Check sheet for the modelled part. Datum: model origin and axes. Units: mm. A direction names the side the tool comes from. Round coordinates to 2 decimals unless told otherwise and drop trailing zeros. Write each loop counter-clockwise with the first axis right and the second up, starting at its lowest first coordinate (ties: lowest second). Pieces come first, ordered by that corner, then holes. Notation, with made-up numbers: M 0,68.5 L 7,68.5 A20 ccw 7,95.5 Z; hole C -1,85.25 d10. An arc over 180 degrees is marked long. Put each result on its own line as item: value.
```python
from build123d import *

# Parameters (mm, degrees)
SKETCH1_W           = 30
SKETCH1_H           = 12
BOSS_EXTRUDE1_DEPTH = 3
SKETCH3_W           = 5
SKETCH3_H           = 3
BOSS_EXTRUDE2_DEPTH = 3
SKETCH4_W           = 3
SKETCH4_H           = 3
CUT_EXTRUDE1_DEPTH  = 10


with BuildPart() as part:
    # Sketch1 → Boss-Extrude1 (new body)
    with BuildSketch(Plane(origin=(0, 0, 0), x_dir=(0, 0, -1), z_dir=(1, 0, 0))):
        Rectangle(SKETCH1_W, SKETCH1_H)
    extrude(amount=BOSS_EXTRUDE1_DEPTH)

    # Sketch3 → Boss-Extrude2 (add)
    with BuildSketch(Plane(origin=(3, 0, 0), x_dir=(0, 0, -1), z_dir=(1, 0, 0))):
        with Locations((-10, 7.5)):
            Rectangle(SKETCH3_W, SKETCH3_H)
        with Locations((0, 7.5)):
            Rectangle(SKETCH3_W, SKETCH3_H)
        with Locations((10, 7.5)):
            Rectangle(SKETCH3_W, SKETCH3_H)
        with Locations((10, -7.5)):
            Rectangle(SKETCH3_W, SKETCH3_H)
        with Locations((0, -7.5)):
            Rectangle(SKETCH3_W, SKETCH3_H)
        with Locations((-10, -7.5)):
            Rectangle(SKETCH3_W, SKETCH3_H)
    extrude(amount=-BOSS_EXTRUDE2_DEPTH)

    # Sketch4 → Cut-Extrude1 (cut)
    with BuildSketch(Plane(origin=(3, 0, 0), x_dir=(0, 0, -1), z_dir=(1, 0, 0))):
        with Locations((-5, -1.5)):
            Rectangle(SKETCH4_W, SKETCH4_H)
        with Locations((5, -1.5)):
            Rectangle(SKETCH4_W, SKETCH4_H)
    extrude(amount=-CUT_EXTRUDE1_DEPTH, mode=Mode.SUBTRACT)


solid = part.part
```
1. Cross-section at D-D (z = 13.25). Enter the section's corners in (x, y), then the cut area to 3 significant figures.
Computed values:
outline: M 0,-6 L 3,-6 L 3,6 L 0,6 Z
area: 36.0 mm2
2. Access from +Z, -Z, +X, -X, +Y, -Y to the whole of each face (thin tool, end or side, straight path). Record for faces 4 (the flat face through (2, 7, 2.5)), 5 (the flat face through (2, -8, -2.5)), 6 (the flat face through (2, -3, 5)), 7 (the flat face through (1, -6, 14)).
Computed values:
face 4: +X, -X, +Y
face 5: +X, -X, -Y
face 6: +X, -X
face 7: +Z, +X, -X, -Y
3. Release check for a two-part mould opening along Z. For faces 1 (the flat face through (2, 0, -5)), 2 (the flat face through (1, -6, -14)), 3 (the flat face through (2, 7, -12.5)) record: +Z half, -Z half, draft (parallel to the pull), parting line (faces both ways), or undercut.
Computed values:
face 1: undercut
face 2: draft
face 3: -Z half
4. Cross-section at C-C (x = 1.05). Count the separate pieces of the cut face and the enclosed holes in it, then the cut area to 3 significant figures.
Computed values:
separate pieces: 1
enclosed holes: 2
area: 432 mm2
5. Scan lines: probe 1 along Z at (x, y) = (0.4, -6.5); probe 2 along Z at (x, y) = (1.1, -2); probe 3 along Y at (x, z) = (2, -4.5). Record each from-to range of solid material in increasing order.
Computed values:
probe 1: z = -12.5 to -7.5, -2.5 to 2.5, 7.5 to 12.5
probe 2: z = -15 to -6.5, -3.5 to 3.5, 6.5 to 15
probe 3: y = -6 to -3, 0 to 6
6. Cross-section at B-B (y = 7.25). Enter the section's corners in (x, z).
Computed values:
outline: M 0,-12.5 L 3,-12.5 L 3,-7.5 L 0,-7.5 Z; M 0,-2.5 L 3,-2.5 L 3,2.5 L 0,2.5 Z; M 0,7.5 L 3,7.5 L 3,12.5 L 0,12.5 Z
7. Depth check by flat-ended pin: pin 1 Ø0.8 at (x, z) = (2, -14) entering from +Y; pin 2 Ø0.9 at (x, y) = (1.5, -8) entering from -Z. Enter the tip coordinate at first touch or a pass-through.
Computed values:
pin 1: stops at y = 6
pin 2: stops at z = -12.5
8. Cross-section at A-A (z = -4.5). Enter the section's corners in (x, y).
Computed values:
outline: M 0,-6 L 3,-6 L 3,-3 L 0,-3 Z; M 0,0 L 3,0 L 3,6 L 0,6 Z
